```python
from build123d import *

# Parameters (mm, degrees)
F1_DEPTH = 9


with BuildPart() as f1:
    # F0 (on Top) → F1 (new body)
    with BuildSketch(Plane.XY):
        with BuildLine():
            Line((-9.846154, -38.769231), (-5, -40))
            Line((-5, -40), (-5, -50))
            Line((-5, -50), (5, -50))
            Line((5, -50), (5, -40))
            Line((5, -40), (9.846154, -38.769231))
            ThreePointArc((9.846154, -38.769231), (24.557625, 31.574089), (-40, 0))
            Line((-40, 0), (-40, -23.162289))
            ThreePointArc((-40, -23.162289), (-41.464466, -26.697823), (-45, -28.162289))
            Line((-45, -28.162289), (-80, -28.162289))
            Line((-80, -28.162289), (-80, -30.753131))
            Line((-80, -30.753131), (-42.426797, -31.917549))
            ThreePointArc((-42.426797, -31.917549), (-32.849773, -29.413912), (-23.420478, -32.426551))
            ThreePointArc((-23.420478, -32.426551), (-16.932944, -36.239142), (-9.846154, -38.769231))
        make_face()
        with BuildLine():
            Line((-38.29699, -23.521098), (-38, 0))
            ThreePointArc((-38, 0), (33.844209, 17.279164), (-22.285815, -30.778929))
            ThreePointArc((-22.285815, -30.778929), (-22.479913, -30.637453), (-22.673113, -30.494753))
            ThreePointArc((-22.673113, -30.494753), (-28.646621, -27.517054), (-35.251991, -26.558634))
            ThreePointArc((-35.251991, -26.558634), (-37.415945, -25.682896), (-38.29699, -23.521098))
        make_face(mode=Mode.SUBTRACT)
    extrude(amount=F1_DEPTH)


solid = f1.part
```
Here's how the part is built. I have some questions about the finished solid (model axes, mm). A direction names the side the tool comes from. Coordinates: 2 decimals unless noted, no trailing zeros. Loops run counter-clockwise (first coordinate to the right, second up) from the corner with the lowest first, then second, coordinate; pieces in that order, holes last. Notation, with made-up numbers: (49.5, 11) - (90.5, 11) arc R26 cw to (90.5, 29) - close; hole circle Ø11 at (8.5, -28.75). An arc over 180 degrees is marked (long way). Return JSON: item names as keys, results as strings. Group by question number.
Item 1: Will these pins go through, and if not, where does the flat tip stop? P1, Ø1, axis at x = -54.5, y = -27, coming from the +Z side; P2, Ø1.5, axis at x = -67, z = 2, coming from the -Y side; P3, Ø5, axis at y = -4.5, z = 8, coming from the +X side; P4, Ø2.5, axis at y = -43.5, z = 3.5, coming from the -X side.
Item 2: If we section it at C-C on z = 5.5: Write out the boundary of the cut face in (x, y), and give its area (3 significant figures).
Item 3: On a 3-axis mill with a long thin cutter (end or side, diameter ignored), from which of +Z, -Z, +X, -X, +Y, -Y can I reach the whole of each face in a straight line? I mean faces 1 (the face through (5, -45, 4)), 2 (the face through (-40, -11, 4)), 3 (the face through (-5, -45, 4)), 4 (the face through (-28.557, -27.545, 4.437)), 5 (the face through (0, -50, 4)). Say none if no direction works.
Item 4: If we section it at A-A on y = 17: Write out the boundary of the cut face in (x, z).
Item 5: If we section it at B-B on x = 0: Write out the boundary of the cut face in (y, z).
Item 6: If we section it at D-D on x = -64.5: Write out the boundary of the cut face in (y, z), and give its area (3 significant figures).
Item 7: I need wall thicknesses on line 1 (Y direction, x = 0, z = 6); line 2 (X direction, y = 0, z = 3.25); line 3 (X direction, y = 9, z = 6.5). Which ranges of each line are inside material? Lowest first, please. Write a range as from..to.
Item 8: We'd pull the mould along Y, two halves only. Please class faces 6 (the face through (-16, -35, 0)), 7 (the face through (33.175, 18.532, 4.437)), 8 (the face through (-32.99, -29.41, 4.44)), 9 (the face through (25.532, 30.791, 4.437)): +Y half, -Y half, draft (parallel to the pull), parting line (faces both ways), or undercut.
Calculated:
{
 "1": {"P1": "passes through", "P2": "stops at y = -31.18", "P3": "stops at x = 39.95", "P4": "stops at x = -5"},
 "2": {"outline": "(-80, -30.75) - (-42.43, -31.92) arc R17.76 cw to (-23.42, -32.43) arc R40 ccw to (-9.85, -38.77) - (-5, -40) - (-5, -50) - (5, -50) - (5, -40) - (9.85, -38.77) arc R40 ccw (long way) to (-40, 0) - (-40, -23.16) arc R5 cw to (-45, -28.16) - (-80, -28.16) - close; hole (-38.3, -23.52) arc R3 ccw to (-35.25, -26.56) arc R21.06 cw to (-22.67, -30.49) arc R38 ccw to (-22.29, -30.78) arc R38 ccw (long way) to (-38, 0) - close", "area": "750 mm^2"},
 "3": {"face 1": "+Z, -Z, +X, -Y", "face 2": "+Z, -Z, -X, +Y", "face 3": "+Z, -Z, -X, -Y", "face 4": "+Z, -Z", "face 5": "+Z, -Z, +X, -X, -Y"},
 "4": {"outline": "(-36.21, 0) - (-33.99, 0) - (-33.99, 9) - (-36.21, 9) - close; (33.99, 0) - (36.21, 0) - (36.21, 9) - (33.99, 9) - close"},
 "5": {"outline": "(-50, 0) - (-38, 0) - (-38, 9) - (-50, 9) - close; (38, 0) - (40, 0) - (40, 9) - (38, 9) - close"},
 "6": {"outline": "(-31.23, 0) - (-28.16, 0) - (-28.16, 9) - (-31.23, 9) - close", "area": "27.6 mm^2"},
 "7": {"line 1": "y = -50..-38, 38..40", "line 2": "x = -40..-38, 38..40", "line 3": "x = -38.97..-36.92, 36.92..38.97"},
 "8": {"face 6": "draft", "face 7": "undercut", "face 8": "-Y half", "face 9": "parting line"}
}
